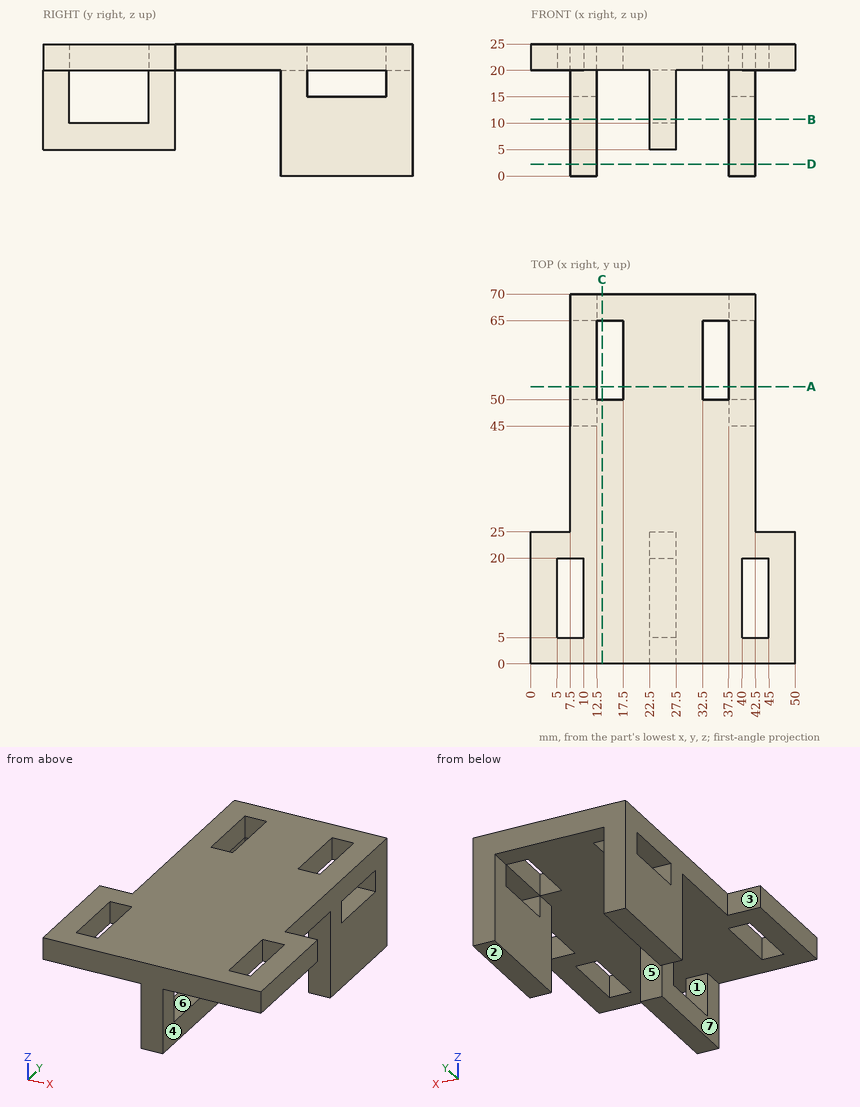
Print and shaded views of the part. All mm, measured from the part's lowest x, y and z. A direction names the side the tool comes from. Coordinates: 2 decimals unless noted, no trailing zeros. Loops run counter-clockwise (first coordinate to the right, second up) from the corner with the lowest first, then second, coordinate; pieces in that order, holes last. Notation, with made-up numbers: (-35, -37.75) - (-3, -37.75) arc R19 ccw to (-3, -14.75) - close; hole circle Ø7 at (33, -18). An arc over 180 degrees is marked (long way). Write item = value, one per line. Start each with the question number.
Item 1: Wall check: probe 1 along X at (y, z) = (48.5, 5.75); probe 2 along Z at (x, y) = (39, 53); probe 3 along Y at (x, z) = (34, 21.75). Give the ranges that are in metal, low to high. Write a range as [from, to].
Item 2: Drop flat-ended pins along their axis: pin 1 Ø12 at (y, z) = (16.5, 13.5) entering from -X; pin 2 Ø2.5 at (y, z) = (61, 23) entering from +X; pin 3 Ø5 at (x, y) = (39.5, 17.5) entering from -Z. Give the stop position or say it passes through.
Item 3: Saw through at C-C, the plane x = 13.5. List the corners of the cut face in (y, z).
Item 4: Saw through at D-D, the plane z = 2.25. List the corners of the cut face in (x, y).
Item 5: Saw through at A-A, the plane y = 52.5. List the corners of the cut face in (x, z).
Item 6: 3-axis set-ups, long thin cutter, end or side, ignore diameter. For the marked faces 4, 5, 6 and 7: which of +Z, -Z, +X, -X, +Y, -Y reach the whole face in a straight line?
Item 7: Pull direction Z, two halves, no side cores. Call the marked faces 1, 2 and 3: +Z half, -Z half, draft (parallel to the pull), parting line (faces both ways), or undercut.
Item 8: Saw through at B-B, the plane z = 10.75. List the corners of the cut face in (x, y), then the cut area to 3 significant figures.
Answers:
q1.probe_1 = [7.5, 12.5], [37.5, 42.5]
q1.probe_2 = [0, 15], [20, 25]
q1.probe_3 = [0, 50], [65, 70]
q2.pin_1 = 22.5
q2.pin_2 = 42.5
q2.pin_3 = 20
q3.outline = (0, 20) - (50, 20) - (50, 25) - (0, 25) - close; (65, 20) - (70, 20) - (70, 25) - (65, 25) - close
q4.outline = (7.5, 45) - (12.5, 45) - (12.5, 70) - (7.5, 70) - close; (37.5, 45) - (42.5, 45) - (42.5, 70) - (37.5, 70) - close
q5.outline = (7.5, 0) - (12.5, 0) - (12.5, 15) - (7.5, 15) - close; (7.5, 20) - (12.5, 20) - (12.5, 25) - (7.5, 25) - close; (17.5, 20) - (32.5, 20) - (32.5, 25) - (17.5, 25) - close; (37.5, 0) - (42.5, 0) - (42.5, 15) - (37.5, 15) - close; (37.5, 20) - (42.5, 20) - (42.5, 25) - (37.5, 25) - close
q6.face_4 = -Z, +X, +Y, -Y
q6.face_5 = -Z, +X, -X, +Y
q6.face_6 = +X, -X
q6.face_7 = -Z, -X, +Y, -Y
q7.face_1 = undercut
q7.face_2 = -Z half
q7.face_3 = draft
q8.outline = (7.5, 45) - (12.5, 45) - (12.5, 70) - (7.5, 70) - close; (22.5, 0) - (27.5, 0) - (27.5, 5) - (22.5, 5) - close; (22.5, 20) - (27.5, 20) - (27.5, 25) - (22.5, 25) - close; (37.5, 45) - (42.5, 45) - (42.5, 70) - (37.5, 70) - close
q8.area = 300 mm2
